Geometry: final body of the model. Coordinates: model frame, mm. A direction names the side the tool comes from. Give positions to 0.01 mm unless a question says otherwise; leave off trailing zeros. Write each loop counter-clockwise with the first axis right and the second up, starting at its lowest first coordinate (ties: lowest second). Pieces come first, ordered by that corner, then holes.
Q1. Section D-D (x = 43.5). Return the cut outline in (y, z), plus the area to 3 significant figures.
Q2. Section B-B (y = 10.5). Return the cut outline in (x, z).
Q3. Section C-C (z = 7.25). Return the cut outline in (x, y).
Q4. Section A-A (x = 7). Return the cut outline in (y, z) (3 decimals).
Q5. Reachability of faces 4 (the cylindrical face through (64.568, 6.632, 2.479)), 5 (the flat face through (72, 7, 0)), 6 (the flat face through (7, 7, 4)) from +Z, -Z, +X, -X, +Y, -Y: full face, straight path, thin tool, end or side. Return the list, or none.
Q6. Line query: line 1 (X direction, y = -1, z = 0); line 2 (Z direction, x = 33.5, y = 8.5); line 3 (Y direction, x = 37.5, z = -1). Output: solid intervals per line, ascending.
Q7. Pin query (flat end, axial travel): pin 1 Ø2.5 at (x, y) = (49.5, 7.5) entering from +Z; pin 2 Ø5 at (x, z) = (51, 4.5) entering from -Y (3 decimals); pin 3 Ø0.9 at (x, z) = (19.5, -1) entering from +Y. Return the tip coordinate at first contact, or that it passes through.
Q8. Mould query, pull axis X, two halves, no side actions, for faces 1 (the cylindrical face through (50.468, 6.632, 2.479)), 2 (the flat face through (34, 0, -1)), 3 (the cylindrical face through (-6.76, 22.01, 17.99)). Classes: +X half, -X half, draft (parallel to the pull), parting line (faces both ways), or undercut.
Autodesk Inventor part; units mm, degrees
ref_plane "YZ Plane" through (0, 0, 0) normal (1, 0, 0) x (0, 1, 0)
ref_plane "XZ Plane" through (0, 0, 0) normal (0, 1, 0) x (-1, 0, 0)
ref_plane "XY Plane" through (0, 0, 0) normal (0, 0, 1) x (1, 0, 0)
sketch "Sketch1" plane through (0, 0, 0) normal (0, 0, 1) x (1, 0, 0)
  line L0 (0, 0) -> (70, 0)
  line L1 (70, 0) -> (70, 14)
  line L2 (70, 14) -> (0, 14)
  line L3 (0, 14) -> (0, 0)
  dimension "d0" = 70
  dimension "d1" = 14
extrude "Extrusion1" add sketch "Sketch1" along normal blind 1
sketch "Sketch2" plane through (0, 0, 1) normal (0, 0, 1) x (1, 0, 0)
  line L0 (70, 14) -> (0, 14)
  line L1 (0, 14) -> (0, 0)
  circle A0 centre (7, 7) radius 1.225
  circle A1 centre (35.2, 7) radius 1.225
  dimension "d5" = 70
  dimension "d6" = 14
  dimension "d9" = 2.45
  dimension "d10" = 2.45
  dimension "d32" = 28.2
extrude "Extrusion5" add sketch "Sketch2" along normal blind 3
sketch "Sketch4" plane through (0, 0, 1) normal (0, 0, 1) x (1, 0, 0)
  circle A0 centre (21.1, 7) radius 2.5
  line L0 (0, 0) -> (70, 0)
  line L1 (0, 14) -> (0, 0)
  circle A1 centre (7, 7) radius 1.225
  point P0 (6, 0)
  point P1 (64, 0)
  point P2 (0, 8)
  point P3 (0, 6)
  dimension "d25" = 5
  dimension "d26" = 7
  dimension "d29" = 14.1
extrude "Extrusion6" add sketch "Sketch4" along normal blind 3 contours A0
sketch "Sketch5" plane through (0, 0, 1) normal (0, 0, 1) x (1, 0, 0)
  circle A0 centre (35.2, 7) radius 1.225
  circle A1 centre (49.3, 7) radius 1.225
  point P0 (0, 0)
  dimension "d34" = 14.1
extrude "Extrusion7" add sketch "Sketch5" along normal blind 3 contours A1
pattern_linear "Rectangular Pattern2" count 2 spacing 14.1 along (1, 0, 0) of "Extrusion7"
sketch "Sketch6" plane through (0, 0, 0) normal (-1, 0, 0) x (0, 0, 1)
  line L0 (1, 0) -> (1, 14)
  line L1 (0, 0) -> (1, 0)
  line L2 (1, 0) -> (1, 14)
  line L3 (1, 14) -> (0, 14)
  line L4 (0, 14) -> (0, 0)
  line L5 (0, 14) -> (1, 14)
  line L6 (0, 0) -> (1, 0)
  line L7 (0, 0) -> (1, 0)
extrude "Extrusion8" add sketch "Sketch6" along normal blind 10
sketch "Sketch7" plane through (-10, 0, 0) normal (-1, 0, 0) x (0, 0, 1)
  line L0 (0, 0) -> (1, 0)
  line L1 (0, 0) -> (1, 0)
  line L2 (1, 0) -> (1, -14)
  line L3 (1, -14) -> (0, -14)
  line L4 (0, -14) -> (0, 0)
  line L5 (0, 13.9913) -> (1, 13.9913)
  line L6 (1, 13.9913) -> (1, 27.9913)
  line L7 (1, 27.9913) -> (0, 27.9913)
  line L8 (0, 27.9913) -> (0, 13.9913)
  line L9 (1, 0) -> (1, 14)
  line L10 (0, 0) -> (0, 14)
  line L11 (1, 14) -> (0, 14)
  line L12 (0, 14) -> (0, 0)
  line L13 (0, 0) -> (1, 0)
  line L14 (1, 0) -> (1, 14)
  dimension "d47" = 14
  dimension "d48" = 14
extrude "Extrusion9" add sketch "Sketch7" against normal blind 7
sketch "Sketch8" plane through (0, 0, 0) normal (0, 0, -1) x (-1, 0, 0)
  line L0 (10, 27.9913) -> (10, -14)
  line L1 (10, 27.9913) -> (3, 27.9913)
  line L2 (3, 27.9913) -> (3, -14)
  line L3 (3, -14) -> (10, -14)
  line L4 (10, -14) -> (10, 27.9913)
  line L5 (-70, 0) -> (-70, 14)
  line L6 (-70, 14) -> (3, 14)
  line L7 (-70, 0) -> (3, 0)
  line L8 (3, 0) -> (3, 14)
  line L9 (3, 14) -> (-70, 14)
  line L10 (-70, 14) -> (-70, 0)
  point P0 (0, 0)
extrude "Extrusion10" add sketch "Sketch8" along normal blind 2
sketch "Sketch9" plane through (0, 0, 1) normal (0, 0, 1) x (1, 0, 0)
  circle A0 centre (-6.5, 23.9913) radius 2
  line L0 (-3, 27.9913) -> (-3, 14)
  line L1 (-10, 27.9913) -> (-3, 27.9913)
  circle A1 centre (-6.5, 6.9913) radius 2
  circle A2 centre (-6.5, -10.0087) radius 2
  line L2 (-10, -14) -> (-3, -14)
  line L3 (-10, -14) -> (-10, 27.9913)
  point P0 (0, 0)
  dimension "d53" = 4
  dimension "d54" = 3.5
  dimension "d55" = 4
  dimension "d58" = 17
  dimension "d63" = 41.9913
  dimension "d64" = 17
  dimension "d65" = 3.9913
extrude "Extrusion11" add sketch "Sketch9" along normal blind 18
sketch "Sketch10" plane through (0, 0, 1) normal (0, 0, 1) x (1, 0, 0)
  line L0 (-10, -14) -> (-3, -14)
  line L1 (-3, 27.9913) -> (-10, 27.9913)
  line L2 (-10, 27.9913) -> (-10, -14)
  line L3 (-10, -14) -> (-3, -14)
  line L4 (-3, -14) -> (-3, 27.9913)
  point P0 (0, 0)
extrude "Extrusion12" add sketch "Sketch10" along normal blind 16
sketch "Sketch11" plane through (70, 0, 1) normal (1, 0, 0) x (0, 0, -1)
  line L0 (3, 0) -> (0, 0)
  line L1 (3, 14) -> (0, 14)
  line L2 (3, 0) -> (0, 0)
  line L3 (0, 0) -> (0, 14)
  line L4 (0, 14) -> (3, 14)
  line L5 (3, 14) -> (3, 0)
  point P0 (1, 0)
extrude "Extrusion13" add sketch "Sketch11" along normal blind 2
properties part number "Kroller Holder2"
Computed:
1. outline: (0, -2) - (14, -2) - (14, 1) - (0, 1) - close
1. area: 42.0 mm2
2. outline: (-10, -2) - (72, -2) - (72, 1) - (-3, 1) - (-3, 17) - (-10, 17) - close
3. outline: (-10, -14) - (-3, -14) - (-3, 27.99) - (-10, 27.99) - close
4. outline: (0, -2) - (14, -2) - (14, 1) - (8.225, 1) - (8.225, 4) - (5.775, 4) - (5.775, 1) - (0, 1) - close
5. face 4: +Z
5. face 5: +Z, -Z, +X, +Y, -Y
5. face 6: +Z, +X, +Y, -Y
6. line 1: x = -10 to -3
6. line 2: z = -2 to 1
6. line 3: y = 0 to 14
7. pin 1: stops at z = 4
7. pin 2: stops at y = 5.775
7. pin 3: stops at y = 14
8. face 1: undercut
8. face 2: draft
8. face 3: parting line
